The listing builds one solid part. Answer for the finished solid, in the listing's coordinates (mm). Coordinates: 2 decimals unless noted, no trailing zeros. Order: outer loops, then holes, each group sorted by start corner. A loop starts at its lowest first (then second) coordinate and runs counter-clockwise, first axis right, second up. Notation, with made-up numbers: (-23.5, 52) -> (5.5, 52) arc R8 ccw to (5.5, 67) -> close; hole circle Ø9 at (6.5, 7.25). An arc over 180 degrees is marked (long way). Return JSON: item names as keys, results as strings.
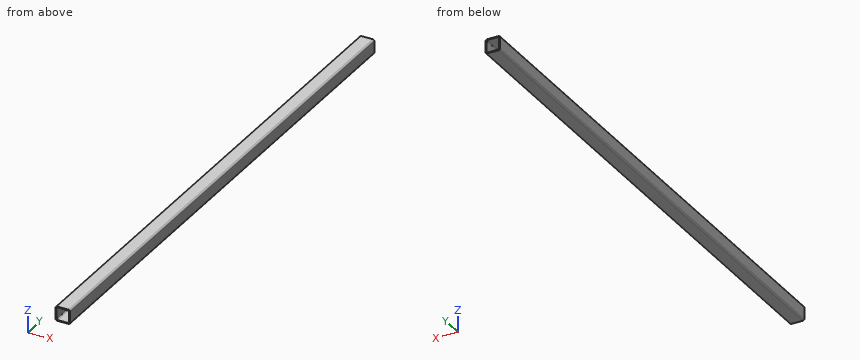
```python
from build123d import *

# Parameters (mm, degrees)
F0_W     = 50
F0_H     = 50
F0_W_2   = 44
F0_H_2   = 44
F1_DEPTH = 1900
F2_DEPTH = 100
F3_R     = 5
F4_R     = 3


with BuildPart() as f1:
    # F0 (on Front) → F1 (new body)
    with BuildSketch(Plane.XZ):
        with Locations((25, 25)):
            Rectangle(F0_W, F0_H)
        with Locations((25, 25)):
            Rectangle(F0_W_2, F0_H_2, mode=Mode.SUBTRACT)
    extrude(amount=F1_DEPTH)

    # F0 (on Front) → F2 (join)
    with BuildSketch(Plane.XZ):
        with Locations((25, 25)):
            Rectangle(F0_W, F0_H)
        with Locations((25, 25)):
            Rectangle(F0_W_2, F0_H_2, mode=Mode.SUBTRACT)
    extrude(amount=F2_DEPTH)

    # F3
    f3_edges = [f1.edges().sort_by_distance(p)[0] for p in [
        (50, -950, 50),
        (50, -950, 0),
        (0, -950, 0),
        (0, -950, 50),
    ]]
    fillet(f3_edges, radius=F3_R)

    # F4
    f4_edges = [f1.edges().sort_by_distance(p)[0] for p in [
        (47, -950, 47),
        (3, -950, 3),
        (3, -950, 47),
        (47, -950, 3),
    ]]
    fillet(f4_edges, radius=F4_R)


solid = f1.part
```
Item 1: The part is cut by section A-A on z = 15.5. Determine the outline of the cut face in (x, y).
Answer list:
{"outline": "(0, -1900) -> (3, -1900) -> (3, 0) -> (0, 0) -> close; (47, -1900) -> (50, -1900) -> (50, 0) -> (47, 0) -> close"}
Item 2: The part is cut by section C-C on x = 23. Determine the outline of the cut face in (y, z), plus the area to 3 significant figures.
Answer list:
{"outline": "(-1900, 0) -> (0, 0) -> (0, 3) -> (-1900, 3) -> close; (-1900, 47) -> (0, 47) -> (0, 50) -> (-1900, 50) -> close", "area": "11,400 mm2"}
Item 3: Find the intervals of material crossed by probe 1 along Z at (x, y) = (40, -1473); probe 2 along Z at (x, y) = (5, -1507), in increasing order.
Answer list:
{"probe 1": "0 to 3, 47 to 50", "probe 2": "0 to 3.17, 46.83 to 50"}
Item 4: Flat-ended cylindrical pins translate along their axes: pin 1 (10 mm diameter, centred on x = 39.5, z = 30.5, fed in from -Y); pin 2 (12 mm diameter, centred on x = 38, z = 44.5, fed in from +Y). Find the tip coordinate at first contact, or state that the pin passes through.
Answer list:
{"pin 1": "through", "pin 2": "y = 0"}
Item 5: The part is cut by section B-B on y = -1184.5. Determine the outline of the cut face in (x, z).
Answer list:
{"outline": "(0, 5) arc R5 ccw to (5, 0) -> (45, 0) arc R5 ccw to (50, 5) -> (50, 45) arc R5 ccw to (45, 50) -> (5, 50) arc R5 ccw to (0, 45) -> close; hole (3, 6) arc R3 ccw to (6, 3) -> (44, 3) arc R3 ccw to (47, 6) -> (47, 44) arc R3 ccw to (44, 47) -> (6, 47) arc R3 ccw to (3, 44) -> close"}
